Study the drawing (mm; zero at the part's minimum x, y, z) and answer. Coordinates: 2 decimals unless noted, no trailing zeros. Order: outer loops, then holes, each group sorted by start corner. A loop starts at its lowest first (then second) coordinate and runs counter-clockwise, first axis right, second up. Notation, with made-up numbers: M -27.75,86.25 L -20.75,86.25 A29 cw -20.75,119.25 Z; hole C 67.5,88 d1. An arc over 180 degrees is marked long. Use a Markdown table: item, result. Add a question column.
1) Each of these flat-tipped pins is pushed along its axis until it touches: pin 1 Ø1.2 at (y, z) = (1.5, 9.5) entering from -X; pin 2 Ø10.5 at (x, z) = (29.5, 8.5) entering from +Y; pin 3 Ø5 at (y, z) = (6, 9) entering from -X. Where does it stop, or does it pass through?
2) Find section A-A on x = 20.95. Write down the section's boundary in (y, z), plus the area to 3 significant figures.
3) Find the intervals of material crossed by probe 1 along X at (y, z) = (1, 8.75); probe 2 along Z at (x, y) = (25, 8.25); probe 3 along Y at (x, z) = (6.9, 1.7), in increasing order. Write a range as [from, to].
4) Find section D-D on y = 8.5. Write down the section's boundary in (x, z).
5) Find section C-C on y = 4. Write down the section's boundary in (x, z), plus the area to 3 significant figures.
6) Find section B-B on z = 16.75. Write down the section's boundary in (x, y), plus the area to 3 significant figures.
7) The mould has two halves that part along Z. Classify the marked faces 1, 2, 3 and 4: released by +Z, released by -Z, zero draft, split by the parting line, or undercut.
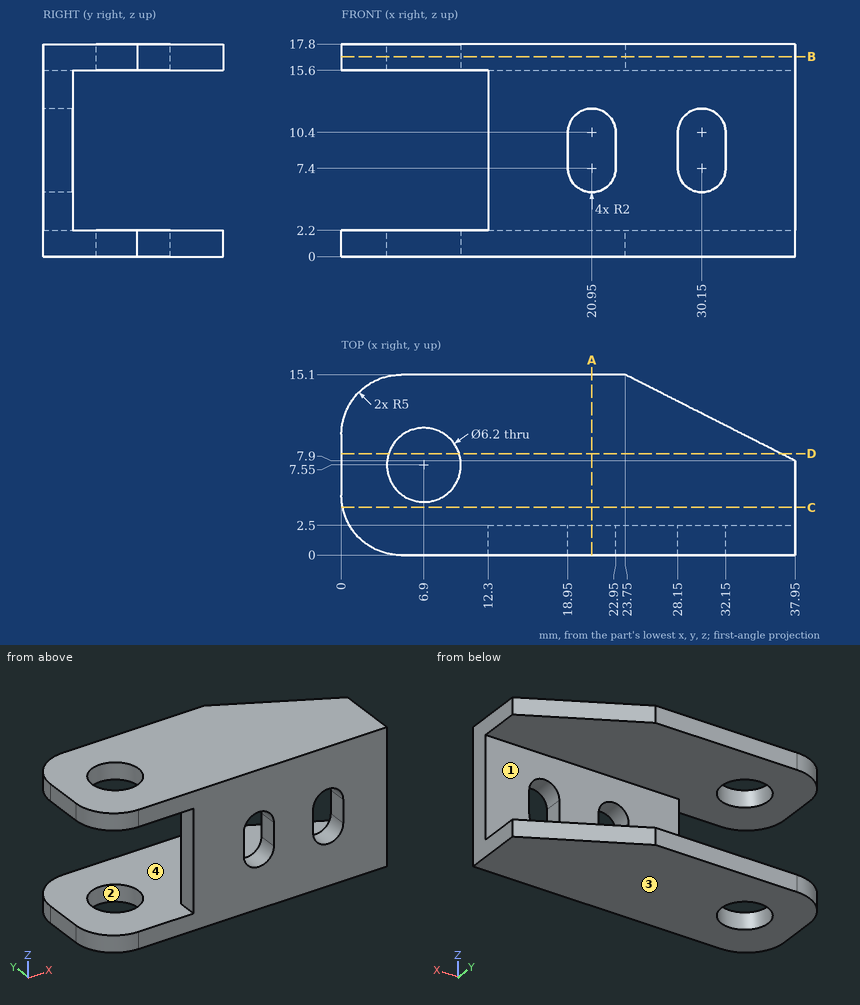
Check result:
| question | item | result |
|---|---|---|
| 1 | pin 1 | stops at x = 12.3 |
| 1 | pin 2 | stops at y = 2.5 |
| 1 | pin 3 | passes through |
| 2 | outline | M 0,0 L 15.1,0 L 15.1,2.2 L 2.5,2.2 L 2.5,5.4 L 0,5.4 Z; M 0,12.4 L 2.5,12.4 L 2.5,15.6 L 15.1,15.6 L 15.1,17.8 L 0,17.8 Z |
| 2 | area | 82.4 mm2 |
| 3 | probe 1 | x = [12.3, 18.95], [22.95, 28.15], [32.15, 37.95] |
| 3 | probe 2 | z = [0, 2.2], [15.6, 17.8] |
| 3 | probe 3 | y = [0, 4.45], [10.65, 15.1] |
| 4 | outline | M 0,0 L 3.95,0 L 3.95,2.2 L 0,2.2 Z; M 0,15.6 L 3.95,15.6 L 3.95,17.8 L 0,17.8 Z; M 9.85,0 L 36.77,0 L 36.77,2.2 L 9.85,2.2 Z; M 9.85,15.6 L 36.77,15.6 L 36.77,17.8 L 9.85,17.8 Z |
| 5 | outline | M 0.1,0 L 37.95,0 L 37.95,2.2 L 0.1,2.2 Z; M 0.1,15.6 L 37.95,15.6 L 37.95,17.8 L 0.1,17.8 Z |
| 5 | area | 167 mm2 |
| 6 | outline | M 0,5 A5 ccw 5,0 L 37.95,0 L 37.95,7.9 L 23.75,15.1 L 5,15.1 A5 ccw 0,10.1 Z; hole C 6.9,7.55 d6.2 |
| 6 | area | 481 mm2 |
| 7 | face 1 | undercut |
| 7 | face 2 | zero draft |
| 7 | face 3 | released by -Z |
| 7 | face 4 | undercut |
